Design review of the part shown in the three views and the two pictorial views. Dimensions are in mm from the part's minimum x, y and z. Give positions to 0.01 mm unless a question says otherwise; leave off trailing zeros. Order: outer loops, then holes, each group sorted by start corner. A loop starts at its lowest first (then second) coordinate and runs counter-clockwise, first axis right, second up.
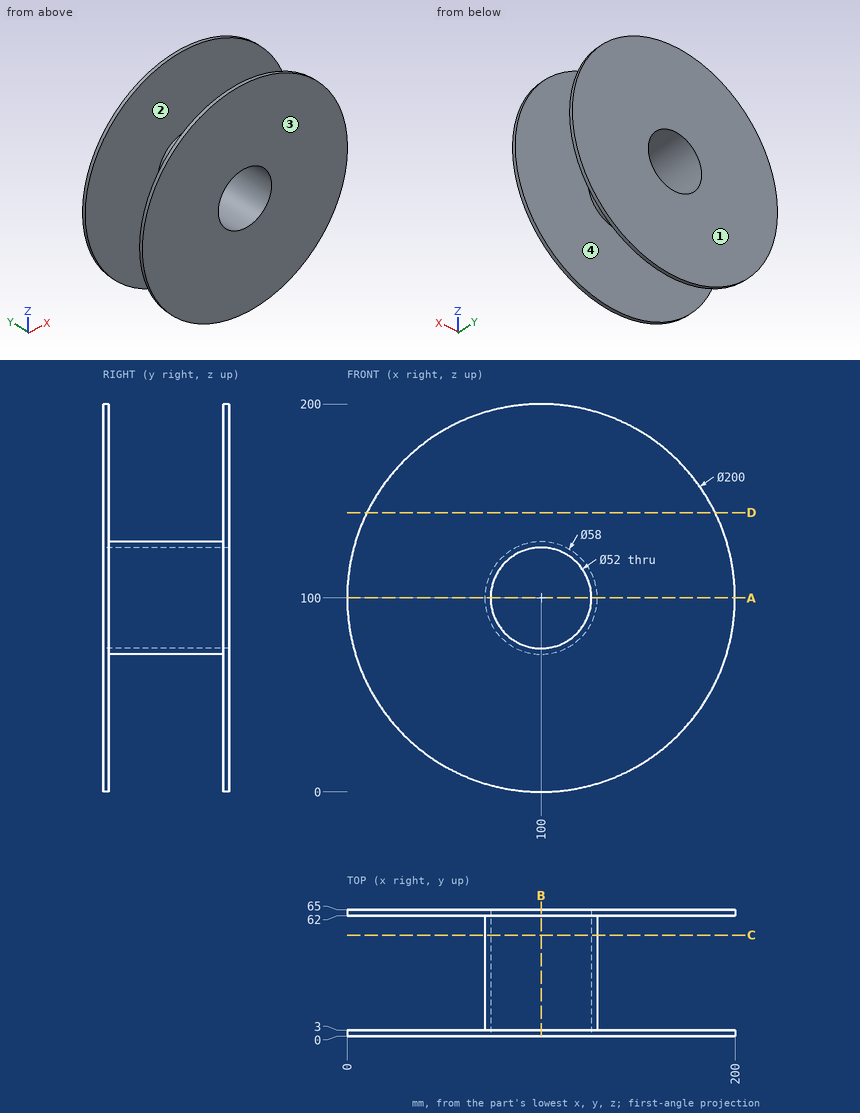
1) We need section D-D on z = 144. Give the boundary of the cut face in (x, y).
Answer sheet:
outline: (10.2, 0) - (189.8, 0) - (189.8, 3) - (10.2, 3) - close; (10.2, 62) - (189.8, 62) - (189.8, 65) - (10.2, 65) - close
2) To check wall thickness, follow line 1 (Y direction, x = 142, z = 78); line 2 (Z direction, x = 100, y = 47.5). State the ranges of each line that lie inside material, in increasing order.
Answer sheet:
line 1: y = 0 to 3, 62 to 65
line 2: z = 71 to 74, 126 to 129
3) Draft analysis for pull direction Y (two halves, no side actions). For the marked faces 1, 2, 3 and 4, state which applies: +Y half, -Y half, draft (parallel to the pull), parting line (faces both ways), or undercut.
Answer sheet:
face 1: +Y half
face 2: undercut
face 3: -Y half
face 4: undercut
4) We need section C-C on y = 52. Give the boundary of the cut face in (x, z), then the cut area to 3 significant figures.
Answer sheet:
outline: circle Ø58 at (100, 100); hole circle Ø52 at (100, 100)
area: 518 mm2
5) We need section B-B on x = 100. Give the boundary of the cut face in (y, z).
Answer sheet:
outline: (0, 0) - (3, 0) - (3, 71) - (62, 71) - (62, 0) - (65, 0) - (65, 74) - (0, 74) - close; (0, 126) - (65, 126) - (65, 200) - (62, 200) - (62, 129) - (3, 129) - (3, 200) - (0, 200) - close
6) We need section A-A on z = 100. Give the boundary of the cut face in (x, y).
Answer sheet:
outline: (0, 0) - (74, 0) - (74, 65) - (0, 65) - (0, 62) - (71, 62) - (71, 3) - (0, 3) - close; (126, 0) - (200, 0) - (200, 3) - (129, 3) - (129, 62) - (200, 62) - (200, 65) - (126, 65) - close
